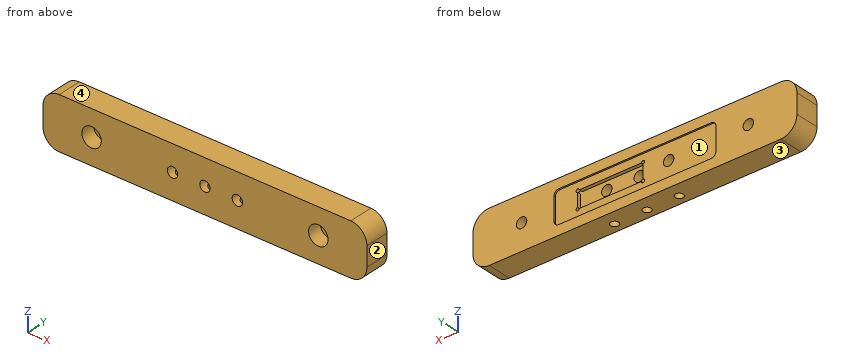
```python
from build123d import *

# Parameters (mm, degrees)
F0_W      = 100
F0_H      = 16
F1_DEPTH  = 7.5
F2_R      = 1.6
F3_DEPTH  = 7.501
F2_R_2    = 3
F4_DEPTH  = 4.4
F5_R      = 1.6
F6_DEPTH  = 7.501
F7_W      = 50
F7_H      = 10
F7_R      = 1.6
F8_DEPTH  = 0.5
F8_FACE_R = 1.6
F9_DEPTH  = 1.6
F10_R     = 1.5
F11_R     = 1.25
F12_DEPTH = 8
F13_R     = 5
F14_DEPTH = 8
F15_DEPTH = 7.501


with BuildPart() as f1:
    # F0 (on Front) → F1 (new body)
    with BuildSketch(Plane.XZ):
        Rectangle(F0_W, F0_H)
    extrude(amount=F1_DEPTH)

    # F2 (on face) → F3 (cut, through all)
    with BuildSketch(Plane.XZ.offset(7.5)):
        with Locations((35, 0)):
            Circle(F2_R)
        with Locations((-35, 0)):
            Circle(F2_R)
    extrude(amount=-F3_DEPTH, mode=Mode.SUBTRACT)

    # F2 (on face) → F4 (cut)
    with BuildSketch(Plane.XZ.offset(7.5)):
        with Locations((35, 0)):
            Circle(F2_R_2)
        with Locations((35, 0)):
            Circle(F2_R, mode=Mode.SUBTRACT)
        with Locations((-35, 0)):
            Circle(F2_R_2)
        with Locations((-35, 0)):
            Circle(F2_R, mode=Mode.SUBTRACT)
    extrude(amount=-F4_DEPTH, mode=Mode.SUBTRACT)

    # F5 (on face) → F6 (cut, through all)
    with BuildSketch(Plane.XZ.offset(7.5)):
        with Locations((10, 0)):
            Circle(F5_R)
        with Locations((-10, 0)):
            Circle(F5_R)
    extrude(amount=-F6_DEPTH, mode=Mode.SUBTRACT)

    # F7 (on face) → F8 (cut)
    with BuildSketch(Plane(origin=(0, 0, 0), x_dir=(-1, 0, 0), z_dir=(0, 1, 0))):
        Rectangle(F7_W, F7_H)
        with BuildLine():
            ThreePointArc((-18.1, 2.1), (-18.453553, 2.953553), (-17.6, 2.6))
            Line((-17.6, 2.6), (1.6, 2.6))
            ThreePointArc((1.6, 2.6), (2.453553, 2.953553), (2.1, 2.1))
            Line((2.1, 2.1), (2.1, -2.1))
            ThreePointArc((2.1, -2.1), (2.453553, -2.953553), (1.6, -2.6))
            Line((1.6, -2.6), (-17.6, -2.6))
            ThreePointArc((-17.6, -2.6), (-18.453553, -2.953553), (-18.1, -2.1))
            Line((-18.1, -2.1), (-18.1, 2.1))
        make_face(mode=Mode.SUBTRACT)
        with Locations((10, 0)):
            Circle(F7_R, mode=Mode.SUBTRACT)
    extrude(amount=-F8_DEPTH, mode=Mode.SUBTRACT)

    # F8_face (on face) → F9 (cut)
    with BuildSketch(Plane(origin=(7.838104, 0, 0), x_dir=(1, 0, 0), z_dir=(0, 1, 0))):
        with BuildLine():
            Line((9.761896, 2.6), (-9.438104, 2.6))
            ThreePointArc((-9.438104, 2.6), (-10.291658, 2.953553), (-9.938104, 2.1))
            Line((-9.938104, 2.1), (-9.938104, -2.1))
            ThreePointArc((-9.938104, -2.1), (-10.291658, -2.953553), (-9.438104, -2.6))
            Line((-9.438104, -2.6), (9.761896, -2.6))
            ThreePointArc((9.761896, -2.6), (10.615449, -2.953553), (10.261896, -2.1))
            Line((10.261896, -2.1), (10.261896, 2.1))
            ThreePointArc((10.261896, 2.1), (10.615449, 2.953553), (9.761896, 2.6))
        make_face()
        with Locations((2.161896, 0)):
            Circle(F8_FACE_R, mode=Mode.SUBTRACT)
    extrude(amount=-F9_DEPTH, mode=Mode.SUBTRACT)

    # F10
    f10_edges = [f1.edges().sort_by_distance(p)[0] for p in [
        (-25, -0.25, 5),
        (-25, -0.25, -5),
        (25, -0.25, -5),
        (25, -0.25, 5),
    ]]
    fillet(f10_edges, radius=F10_R)

    # F11 (on face) → F12 (cut)
    with BuildSketch(Plane(origin=(0, 0, -8), x_dir=(1, 0, 0), z_dir=(0, 0, -1))):
        with Locations((10, 4.5)):
            Circle(F11_R)
        with Locations((0, 4.5)):
            Circle(F11_R)
    extrude(amount=-F12_DEPTH, mode=Mode.SUBTRACT)

    # F13
    f13_edges = [f1.edges().sort_by_distance(p)[0] for p in [
        (-50, -3.75, 8),
        (-50, -3.75, -8),
        (50, -3.75, 8),
        (50, -3.75, -8),
    ]]
    fillet(f13_edges, radius=F13_R)

    # F11 (on face) → F14 (cut)
    with BuildSketch(Plane(origin=(0, 0, -8), x_dir=(1, 0, 0), z_dir=(0, 0, -1))):
        with Locations((10, 4.5)):
            Circle(F11_R)
        with Locations((0, 4.5)):
            Circle(F11_R)
        with Locations((-10, 4.5)):
            Circle(F11_R)
    extrude(amount=-F14_DEPTH, mode=Mode.SUBTRACT)

    # F5 (on face) → F15 (cut, through all)
    with BuildSketch(Plane.XZ.offset(7.5)):
        with Locations((10, 0)):
            Circle(F5_R)
        with Locations((-10, 0)):
            Circle(F5_R)
        Circle(F5_R)
    extrude(amount=-F15_DEPTH, mode=Mode.SUBTRACT)


solid = f1.part
```
Input: part model. Units: mm. Frame: model coordinates. Face numbers are marked on the shaded views. Coordinates: 2 decimals unless noted, no trailing zeros. Order: outer loops, then holes, each group sorted by start corner. A loop starts at its lowest first (then second) coordinate and runs counter-clockwise, first axis right, second up. Notation, with made-up numbers: (12, 55) - (56, 55) arc R22 ccw to (56, 87) - close; hole circle Ø2 at (19.5, 8). An arc over 180 degrees is marked (long way). Put each result on its own line as item: value.
1. Cut plane C-C on y = -4.5. Return the cut outline in (x, z).
Report:
outline: (-50, -3) arc R5 ccw to (-45, -8) - (-11.25, -8) - (-11.25, -1) arc R1.6 cw (long way) to (-8.75, -1) - (-8.75, -8) - (-1.25, -8) - (-1.25, -1) arc R1.6 cw (long way) to (1.25, -1) - (1.25, -8) - (8.75, -8) - (8.75, -1) arc R1.6 cw (long way) to (11.25, -1) - (11.25, -8) - (45, -8) arc R5 ccw to (50, -3) - (50, 3) arc R5 ccw to (45, 8) - (-45, 8) arc R5 ccw to (-50, 3) - close; hole circle Ø6 at (-35, 0); hole circle Ø6 at (35, 0)
2. Cut plane A-A on x = -35. Return the cut outline in (y, z), then the cut area to 3 significant figures.
Report:
outline: (-7.5, -8) - (0, -8) - (0, -1.6) - (-3.1, -1.6) - (-3.1, -3) - (-7.5, -3) - close; (-7.5, 3) - (-3.1, 3) - (-3.1, 1.6) - (0, 1.6) - (0, 8) - (-7.5, 8) - close
area: 83.7 mm2
3. Cut plane D-D on x = -10. Return the cut outline in (y, z), then the cut area to 3 significant figures.
Report:
outline: (-7.5, -8) - (-5.75, -8) - (-5.75, -1.6) - (-7.5, -1.6) - close; (-7.5, 1.6) - (-0.5, 1.6) - (-0.5, 5) - (0, 5) - (0, 8) - (-7.5, 8) - close; (-3.25, -8) - (0, -8) - (0, -5) - (-0.5, -5) - (-0.5, -1.6) - (-3.25, -1.6) - close
area: 76.6 mm2
4. Contact query for flat-ended pins moving along their axis: pin 1 Ø5 at (x, z) = (12.5, 1.5) entering from +Y; pin 2 Ø0.9 at (x, z) = (-2.1, -2.6) entering from +Y; pin 3 Ø1.8 at (x, z) = (35.5, 1.5) entering from -Y. Output: stop coordinate, or through.
Report:
pin 1: stops at y = -0.5
pin 2: stops at y = -1.6
pin 3: stops at y = -3.1
5. Line query: line 1 along X through (y, z) = (-1, 2.5); line 2 along Y through (x, z) = (0, -4.25); line 3 along Z through (x, y) = (-36, -2). Output: solid intervals per line, ascending.
Report:
line 1: x = -50 to -2.59, 18.59 to 50
line 2: y = -7.5 to -5.75, -3.25 to -0.5
line 3: z = -8 to -1.25, 1.25 to 8
6. Cut plane B-B on z = -6. Return the cut outline in (x, y), then the cut area to 3 significant figures.
Report:
outline: (-49, -7.5) - (49, -7.5) - (49, 0) - (-49, 0) - close; hole circle Ø2.5 at (-10, -4.5); hole circle Ø2.5 at (0, -4.5); hole circle Ø2.5 at (10, -4.5)
area: 720 mm2
7. Draft query along Z for the marked faces 1, 2, 3 and 4. Return one class per face: pulls with the +Z half, pulls with the -Z half, needs draft (parallel to the pull), parting line crosses it, or undercut.
Report:
face 1: undercut
face 2: needs draft
face 3: pulls with the -Z half
face 4: pulls with the +Z half
